Could you check a few things on this drawing? It's one solid part, dimensions in mm from its lowest x, y, z. Coordinates: 2 decimals unless noted, no trailing zeros. Order: outer loops, then holes, each group sorted by start corner. A loop starts at its lowest first (then second) coordinate and runs counter-clockwise, first axis right, second up.
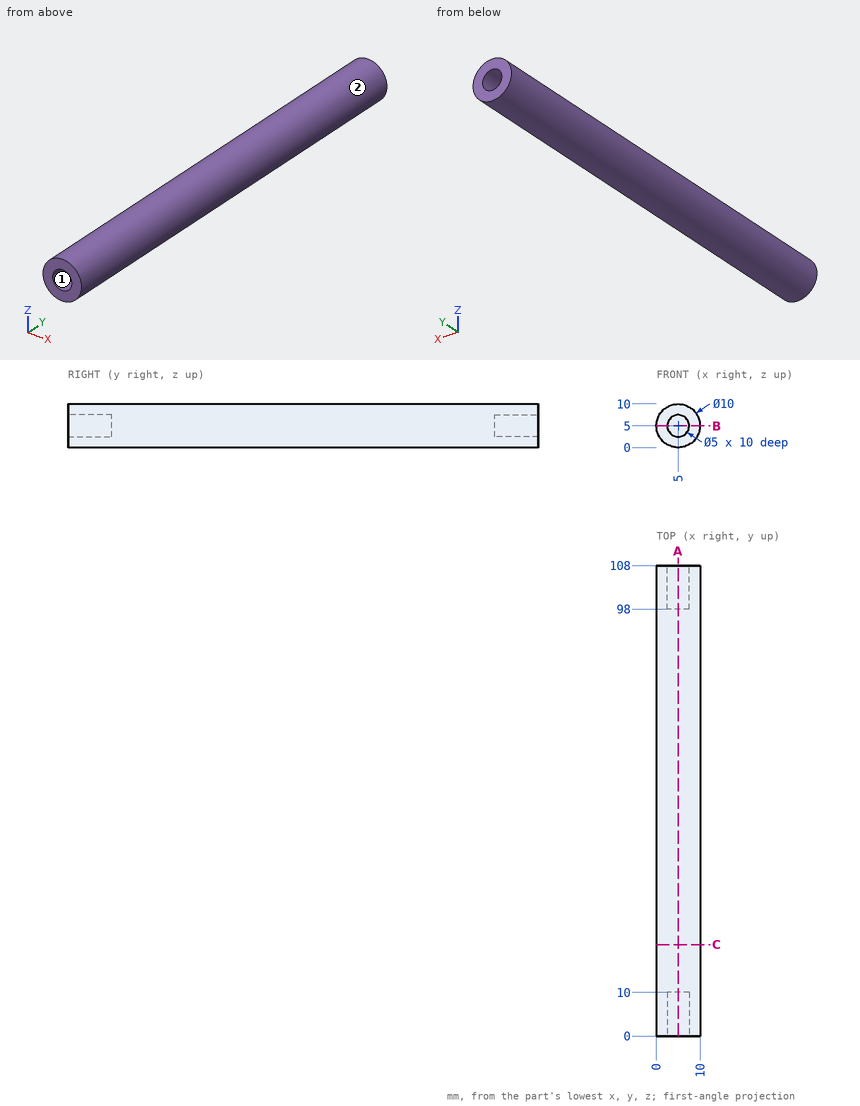
1. Imagine slicing it at C-C on y = 21. Please give me the cut outline in (x, z), then the cut area to 3 significant figures.
Completed:
outline: circle Ø10 at (5, 5)
area: 78.5 mm2
2. Please list where these lines run through material, in increasing order: probe 1 along X at (y, z) = (101.75, 5); probe 2 along Y at (x, z) = (5, 6.5); probe 3 along Z at (x, y) = (4, 46).
Completed:
probe 1: x = 0 to 2.5, 7.5 to 10
probe 2: y = 10 to 98
probe 3: z = 0.1 to 9.9
3. I'm going to push flat-ended pins straight in: pin 1 (4 mm diameter, centred on x = 5, z = 5, fed in from -Y); pin 2 (2.5 mm diameter, centred on x = 4, z = 5.5, fed in from +Y); pin 3 (1.5 mm diameter, centred on x = 1.5, y = 51.5, fed in from +Z). Where does each tip first touch, or does it pass through?
Completed:
pin 1: stops at y = 10
pin 2: stops at y = 98
pin 3: stops at z = 9.18
4. Thinking about a two-plate mould opening in Z: for the marked faces 1 and 2, which applies, pulls with the +Z half, pulls with the -Z half, needs draft (parallel to the pull), parting line crosses it, or undercut?
Completed:
face 1: undercut
face 2: parting line crosses it
5. Imagine slicing it at A-A on x = 5. Please give me the cut outline in (y, z), then the cut area to 3 significant figures.
Completed:
outline: (0, 0) - (108, 0) - (108, 2.5) - (98, 2.5) - (98, 7.5) - (108, 7.5) - (108, 10) - (0, 10) - (0, 7.5) - (10, 7.5) - (10, 2.5) - (0, 2.5) - close
area: 980 mm2
6. Imagine slicing it at B-B on z = 5. Please give me the cut outline in (x, y), then the cut area to 3 significant figures.
Completed:
outline: (0, 0) - (2.5, 0) - (2.5, 10) - (7.5, 10) - (7.5, 0) - (10, 0) - (10, 108) - (7.5, 108) - (7.5, 98) - (2.5, 98) - (2.5, 108) - (0, 108) - close
area: 980 mm2
